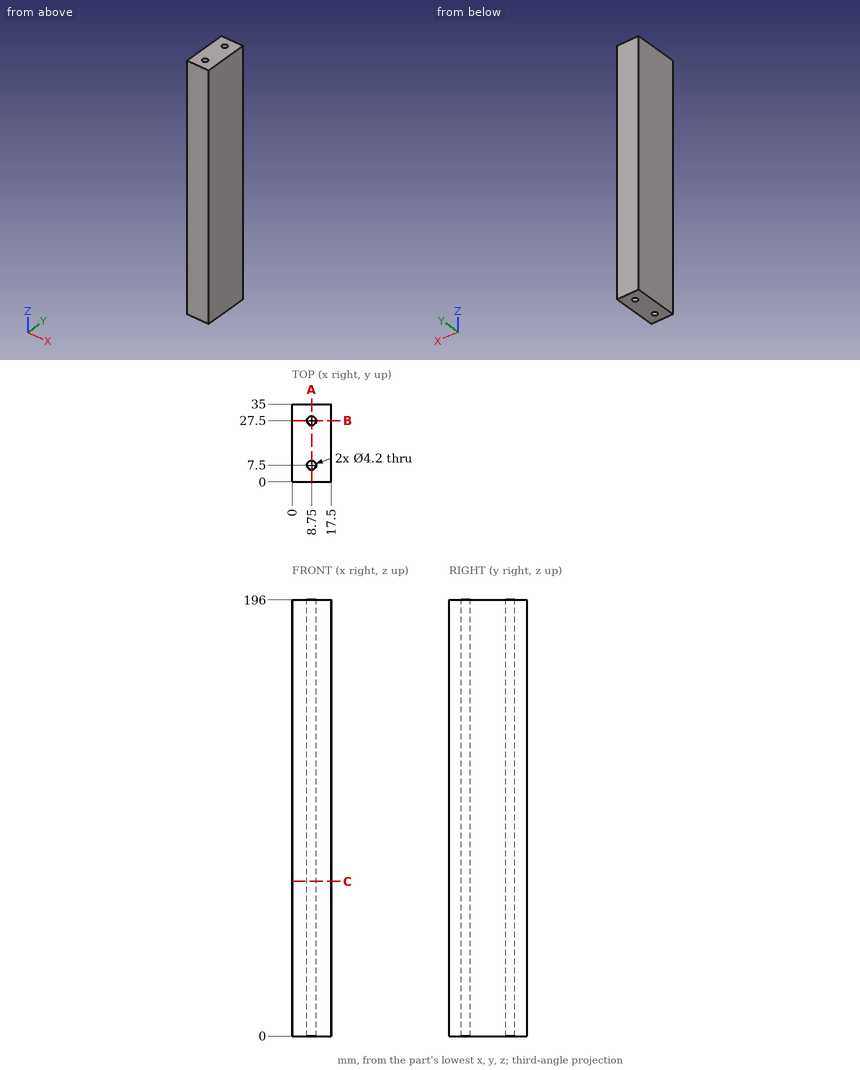
Here's the drawing with two shaded views (mm, measured from the low corner). I have some questions. Give positions to 0.01 mm unless a question says otherwise; leave off trailing zeros. Write each loop counter-clockwise with the first axis right and the second up, starting at its lowest first coordinate (ties: lowest second). Pieces come first, ordered by that corner, then holes. Notation, with made-up numbers: (65, -27) - (117, -27) arc R15 ccw to (117, 2) - close; hole circle Ø2 at (7, 8.5). An arc over 180 degrees is marked (long way). Write item = value, one per line. Start each with the question number.
1. Imagine slicing it at C-C (z = 69.5). Please give me the cut outline in (x, y), and give its area (3 significant figures).
2. Imagine slicing it at A-A (x = 8.75). Please give me the cut outline in (y, z), and give its area (3 significant figures).
3. Please list where these lines run through material, in increasing order: line 1 (Y direction, x = 8.75, z = 149); line 2 (X direction, y = 7.5, z = 159.5); line 3 (Y direction, x = 7.25, z = 48.5).
4. Imagine slicing it at B-B (y = 27.5). Please give me the cut outline in (x, z).
5. For pin 1 (4 mm diameter, centred on x = 8.75, y = 27.5, fed in from -Z), with a flat end and sliding along its axis, tell me the tip position at first contact or that it passes through.
Worked answers:
q1.outline = (0, 0) - (17.5, 0) - (17.5, 35) - (0, 35) - close; hole circle Ø4.2 at (8.75, 7.5); hole circle Ø4.2 at (8.75, 27.5)
q1.area = 585 mm2
q2.outline = (0, 0) - (5.4, 0) - (5.4, 196) - (0, 196) - close; (9.6, 0) - (25.4, 0) - (25.4, 196) - (9.6, 196) - close; (29.6, 0) - (35, 0) - (35, 196) - (29.6, 196) - close
q2.area = 5,210 mm2
q3.line_1 = 0 to 5.4, 9.6 to 25.4, 29.6 to 35
q3.line_2 = 0 to 6.65, 10.85 to 17.5
q3.line_3 = 0 to 6.03, 8.97 to 26.03, 28.97 to 35
q4.outline = (0, 0) - (6.65, 0) - (6.65, 196) - (0, 196) - close; (10.85, 0) - (17.5, 0) - (17.5, 196) - (10.85, 196) - close
q5.pin_1 = through
